Part print with two shaded views. Sizes in mm from the minimum x, y, z corner. A direction names the side the tool comes from. Give positions to 0.01 mm unless a question says otherwise; leave off trailing zeros. Order: outer loops, then holes, each group sorted by start corner. A loop starts at its lowest first (then second) coordinate and runs counter-clockwise, first axis right, second up. Notation, with made-up numbers: (7.5, 0) -> (25.5, 0) arc R18 ccw to (25.5, 19) -> close; hole circle Ø7 at (58, 61.5). An arc over 180 degrees is marked (long way). Write item = value, one per line. Start each with the question number.
Item 1: Drill centre lines: line 1 along Y through (x, z) = (0.4, 5.5); line 2 along Z through (x, y) = (1.3, 4.25); line 3 along Z through (x, y) = (0.5, 9.25). Where is each one in solid material? Low to high.
Item 2: Tool access for the marked faces 1 and 2: list every direction of +Z, -Z, +X, -X, +Y, -Y with a clear straight run to the whole face (end or side of a thin tool).
Item 3: Band-saw the part on B-B on x = 0.5. Write the cut outline in (y, z), plus the area to 3 significant figures.
Item 4: Pull direction Y, two halves, no side cores. Call the marked faces 3, 4 and 5: +Y half, -Y half, draft (parallel to the pull), parting line (faces both ways), or undercut.
Item 5: Band-saw the part on A-A on z = 4. Write the cut outline in (x, y), plus the area to 3 significant figures.
Item 6: Flat gauge pin, fed straight in: P1, Ø0.8, axis at x = 0.5, y = 8, coming from the -Z side. Where does the tip first touch, or does it go through?
Item 7: Band-saw the part on C-C on y = 6.5. Write the cut outline in (x, z).
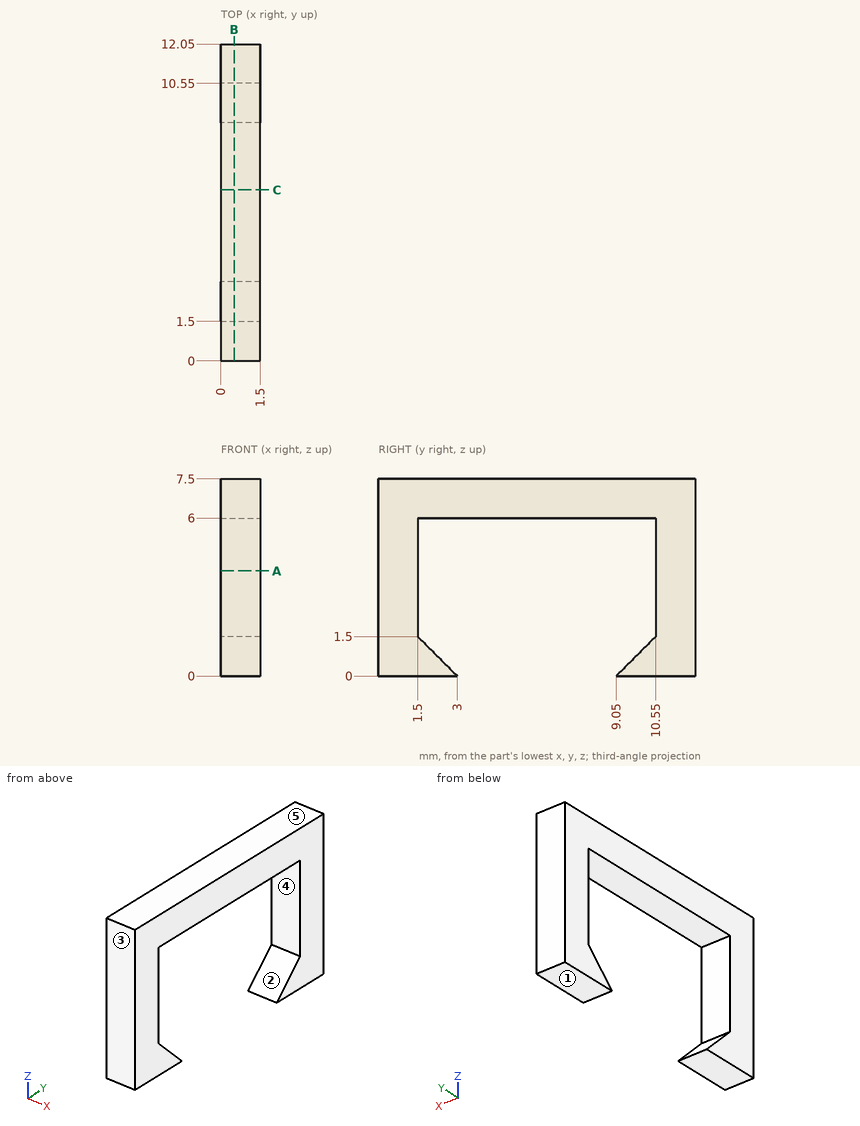
Values found:
q1.line_1 = 0 to 1.5, 10.55 to 12.05
q1.line_2 = 6 to 7.5
q1.line_3 = 0 to 0.2, 6 to 7.5
q2.face_1 = -Z, +X, -X, +Y, -Y
q2.face_2 = +X, -X
q3.outline = (0, 0) -> (3, 0) -> (1.5, 1.5) -> (1.5, 6) -> (10.55, 6) -> (10.55, 1.5) -> (9.05, 0) -> (12.05, 0) -> (12.05, 7.5) -> (0, 7.5) -> close
q3.area = 38.3 mm^2
q4.face_3 = -Y half
q4.face_4 = undercut
q4.face_5 = draft
q5.outline = (0, 0) -> (1.5, 0) -> (1.5, 1.5) -> (0, 1.5) -> close; (0, 10.55) -> (1.5, 10.55) -> (1.5, 12.05) -> (0, 12.05) -> close
q5.area = 4.50 mm^2
q6.P1 = 6
q7.outline = (0, 6) -> (1.5, 6) -> (1.5, 7.5) -> (0, 7.5) -> close
